from build123d import *

# Parameters (mm, degrees)
EXTRUDE_THIN2_DEPTH  = 50
SKETCH3_R            = 10
BOSS_EXTRUDE7_DEPTH  = 45
SKETCH8_R            = 10
BOSS_EXTRUDE8_DEPTH  = 45
SKETCH9_R            = 15
BOSS_EXTRUDE9_DEPTH  = 5
SKETCH10_R           = 15
BOSS_EXTRUDE10_DEPTH = 5


with BuildPart() as part:
    # Sketch1 → Extrude-Thin2 (new body)
    with BuildSketch(Plane.XY):
        with BuildLine():
            Line((-106.417898558, 35), (-106.417898558, 10))
            ThreePointArc((-106.417898558, 10), (-103.48896637, 2.928932188), (-96.417898558, 0))
            Line((-96.417898558, 0), (93.582101442, 0))
            ThreePointArc((93.582101442, 0), (100.653169254, 2.928932188), (103.582101442, 10))
            Line((103.582101442, 10), (103.582101442, 35))
            Line((103.582101442, 35), (113.582101442, 35))
            Line((113.582101442, 35), (113.582101442, 10))
            ThreePointArc((113.582101442, 10), (107.724237066, -4.142135624), (93.582101442, -10))
            Line((93.582101442, -10), (-96.417898558, -10))
            ThreePointArc((-96.417898558, -10), (-110.560034182, -4.142135624), (-116.417898558, 10))
            Line((-116.417898558, 10), (-116.417898558, 35))
            Line((-116.417898558, 35), (-106.417898558, 35))
        make_face()
    extrude(amount=EXTRUDE_THIN2_DEPTH)

    # Sketch3 → Boss-Extrude7 (add)
    with BuildSketch(Plane(origin=(113.582101442, 0, 0), x_dir=(0, 0, -1), z_dir=(1, 0, 0))):
        with Locations((-25, 10)):
            Circle(SKETCH3_R)
    extrude(amount=BOSS_EXTRUDE7_DEPTH)

    # Sketch8 → Boss-Extrude8 (add)
    with BuildSketch(Plane.ZY.offset(116.417898558)):
        with Locations((25, 10)):
            Circle(SKETCH8_R)
    extrude(amount=BOSS_EXTRUDE8_DEPTH)

    # Sketch9 → Boss-Extrude9 (add)
    with BuildSketch(Plane.ZY.offset(116.417898558)):
        with Locations((25, 10)):
            Circle(SKETCH9_R)
    extrude(amount=BOSS_EXTRUDE9_DEPTH)

    # Sketch10 → Boss-Extrude10 (add)
    with BuildSketch(Plane(origin=(113.582101442, 0, 0), x_dir=(0, 0, -1), z_dir=(1, 0, 0))):
        with Locations((-25, 10)):
            Circle(SKETCH10_R)
    extrude(amount=BOSS_EXTRUDE10_DEPTH)


solid = part.part
Work out the finished part from the listing and answer in its coordinate system (mm). A direction names the side the tool comes from. Give positions to 0.01 mm unless a question says otherwise; leave off trailing zeros. Order: outer loops, then holes, each group sorted by start corner. A loop starts at its lowest first (then second) coordinate and runs counter-clockwise, first axis right, second up. Notation, with made-up numbers: (45, 68.25) - (75, 68.25) arc R17 cw to (75, 99.25) - close; hole circle Ø3 at (43.25, -12). An arc over 180 degrees is marked (long way). Answer as CSV lines item,"result". Start each with the question number.
Q1. Given pin 1 Ø12.5 at (y, z) = (26, 13.5) entering from +X; pin 2 Ø2 at (x, y) = (-126.5, 8.5) entering from +Z; pin 3 Ø3 at (x, z) = (-76.5, 41.5) entering from +Y, each flat-ended and moving along its own axis, determine where each tip first touches the part or whether it passes through.
Q2. Find the intervals of material crossed by L1, parallel to X at y = 27, z = 39; L2, parallel to X at y = 24.5, z = 24; L3, parallel to X at y = 1.5, z = 19, in increasing order. Write a range as [from, to].
Q3. The part is cut by section C-C (x = -75.5). Write down the section's boundary in (y, z).
Q4. The mould has two halves that part along X. Classify faces 1 (the face through (-110.4, -4.3, 24.6)), 2 (the face through (158.582, 10, 25)), 3 (the face through (0, -10, 25)): +X half, -X half, draft (parallel to the pull), parting line (faces both ways), or undercut.
Q5. The part is cut by section D-D (z = 30). Write down the section's boundary in (x, y), then the cut area to 3 significant figures.
Q6. The part is cut by section B-B (z = 46). Write down the section's boundary in (x, y).
Q7. The part is cut by section A-A (y = 14). Write down the section's boundary in (x, z).
Q8. For faces 4 (the face through (118.582, 0, 22)), 5 (the face through (-116.418, 28, 25)), 6 (the face through (-118.883, 24.872, 23.047)), 7 (the face through (100.575, 2.852, 24.65)), determine the directions among +Z, -Z, +X, -X, +Y, -Y from which every point of the face is accessible in a straight line to the end or side of a thin tool.
Check result:
1,pin 1,"stops at x = 118.58"
1,pin 2,"stops at z = 34.99"
1,pin 3,"stops at y = 0"
2,L1,"x = [-116.42, -106.42], [103.58, 113.58]"
2,L2,"x = [-121.42, -106.42], [103.58, 118.58]"
2,L3,"x = [-121.42, -116.42], [-114.52, -101.69], [98.85, 111.69], [113.58, 118.58]"
3,outline,"(-10, 0) - (0, 0) - (0, 50) - (-10, 50) - close"
4,face 1,"undercut"
4,face 2,"+X half"
4,face 3,"draft"
5,outline,"(-161.42, 1.34) - (-121.42, 1.34) - (-121.42, -4.14) - (-116.42, -4.14) - (-116.42, 10) arc R20 ccw to (-96.42, -10) - (93.58, -10) arc R20 ccw to (113.58, 10) - (113.58, -4.14) - (118.58, -4.14) - (118.58, 1.34) - (158.58, 1.34) - (158.58, 18.66) - (118.58, 18.66) - (118.58, 24.14) - (113.58, 24.14) - (113.58, 35) - (103.58, 35) - (103.58, 10) arc R10 cw to (93.58, 0) - (-96.42, 0) arc R10 cw to (-106.42, 10) - (-106.42, 35) - (-116.42, 35) - (-116.42, 24.14) - (-121.42, 24.14) - (-121.42, 18.66) - (-161.42, 18.66) - close"
5,area,"4,540 mm²"
6,outline,"(-116.42, 10) arc R20 ccw to (-96.42, -10) - (93.58, -10) arc R20 ccw to (113.58, 10) - (113.58, 35) - (103.58, 35) - (103.58, 10) arc R10 cw to (93.58, 0) - (-96.42, 0) arc R10 cw to (-106.42, 10) - (-106.42, 35) - (-116.42, 35) - close"
7,outline,"(-161.42, 15.83) - (-121.42, 15.83) - (-121.42, 10.54) - (-116.42, 10.54) - (-116.42, 0) - (-106.42, 0) - (-106.42, 50) - (-116.42, 50) - (-116.42, 39.46) - (-121.42, 39.46) - (-121.42, 34.17) - (-161.42, 34.17) - close; (103.58, 0) - (113.58, 0) - (113.58, 10.54) - (118.58, 10.54) - (118.58, 15.83) - (158.58, 15.83) - (158.58, 34.17) - (118.58, 34.17) - (118.58, 39.46) - (113.58, 39.46) - (113.58, 50) - (103.58, 50) - close"
8,face 4,"+X"
8,face 5,"-X, +Y"
8,face 6,"-X"
8,face 7,"+Z, -Z, +Y"
